Read the model definition and answer for the solid it produces. Units are mm, in the model's axes. Face numbers are marked on the shaded views. A direction names the side the tool comes from. Round coordinates to 2 decimals unless told otherwise and drop trailing zeros. Write each loop counter-clockwise with the first axis right and the second up, starting at its lowest first coordinate (ties: lowest second). Pieces come first, ordered by that corner, then holes. Notation, with made-up numbers: (62.5, -8.5) - (89.5, -8.5) arc R14 cw to (89.5, 0.5) - close; hole circle Ø1 at (17, -12). An arc over 180 degrees is marked (long way). Answer as CSV lines item,"result". Start each with the question number.
1) Find section A-A on x = -2. Determine the outline of the cut face in (y, z), then the cut area to 3 significant figures.
2) Which of the six approach directions +Z, -Z, +X, -X, +Y, -Y give full straight-line access (tool end or side, diameter ignored) to the marked faces 1 and 2?
3) Each of these flat-tipped pins is pushed along its axis until it touches: pin 1 (5.5 mm diameter, centred on x = 21.04, z = 663.49, fed in from -Y); pin 2 (2.5 mm diameter, centred on y = 33.5, z = 640, fed in from -X); pin 3 (2 mm diameter, centred on x = -23.5, z = -74.5, fed in from +Y); pin 4 (4.5 mm diameter, centred on x = -21.04, z = 663.49, fed in from +Y). Where does it stop, or does it pass through?
4) Consider line 1 along Y through (x, z) = (14, 189.5); line 2 along Y through (x, z) = (-27, 585); line 3 along Z through (x, y) = (-16.5, 13). Determine where each line is inside the solid, lowest interval first.
5) Find section B-B on z = -339. Determine the outline of the cut face in (x, y), then the cut area to 3 significant figures.
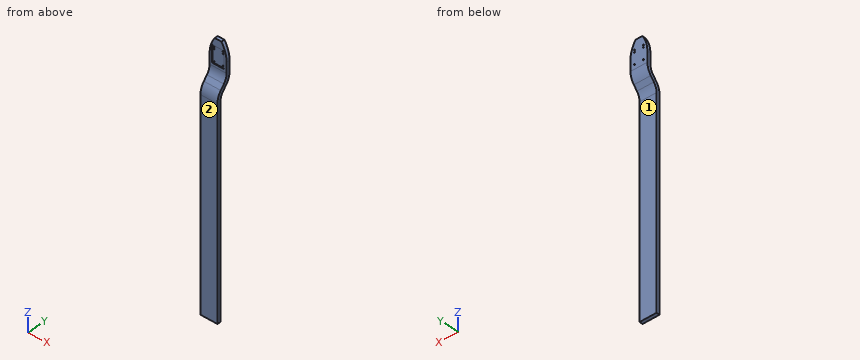
Autodesk Inventor part; units mm, degrees
ref_plane "YZ Plane" through (0, 0, 0) normal (1, 0, 0) x (0, 1, 0)
ref_plane "XZ Plane" through (0, 0, 0) normal (0, 1, 0) x (-1, 0, 0)
ref_plane "XY Plane" through (0, 0, 0) normal (0, 0, 1) x (1, 0, 0)
sketch "Sketch1" plane through (0, 0, 0) normal (0, 1, 0) x (-1, 0, 0)
  line L0 (-40, 482.6) -> (-40, -482.6)
  line L1 (-40, -482.6) -> (40, -482.6)
  line L2 (40, -482.6) -> (40, 482.6)
  line L3 (40, 482.6) -> (-40, 482.6)
  line L4 (-40, 482.6) -> (40, -482.6) construction
  line L5 (-40, -482.6) -> (40, 482.6) construction
  point P0 (0, 0)
  dimension "d0" = 965.2
  dimension "d1" = 80
extrude "Extrusion1" add sketch "Sketch1" against normal blind 15.5448
ref_plane "Work Plane1" through (0, 0, 482.6) normal (1, 0, 0) x (0, 1, 0)
sketch "Sketch2" plane through (0, 0, 482.6) normal (1, 0, 0) x (0, 1, 0)
  line L0 (0, -965.2) -> (0, 0)
  line L1 (0, -965.2) -> (-15.5448, -965.2)
  line L2 (-15.5448, 0) -> (-15.5448, -965.2)
  line L3 (0, 0) -> (-15.5448, 0)
  line L4 (41.9902, -1050.1493) -> (41.9902, -1135.1493)
  line L5 (57.0671, -1050.1493) -> (57.0671, -1135.1493)
  line L6 (57.0671, -1135.1493) -> (41.9902, -1135.1493)
  line L7 (41.9902, -1092.6493) -> (57.0671, -1092.6493) construction
  line L8 (-15.5448, 0) -> (-15.5448, -965.2) construction
  line L9 (-15.5448, -965.2) -> (-15.5448, -1004.6981) construction
  line L10 (-15.5448, -1004.6981) -> (41.9902, -1021.6042) construction
  line L11 (41.9902, -1021.6042) -> (41.9902, -1050.1493) construction
  spline S0 degree 3 poles (-15.5448, -965.2) (-15.5448, -1004.6981) (41.9902, -1021.6042) (41.9902, -1050.1493) knots 1 1 1 1 2 2 2 2
  line L12 (57.0671, -1050.1493) -> (57.0671, -1021.6042) construction
  line L13 (57.0671, -1021.6042) -> (0, -1003.1803) construction
  line L14 (0, -965.2) -> (0, 0) construction
  line L15 (0, -1003.1803) -> (0, -965.2) construction
  spline S1 degree 3 poles (57.0671, -1050.1493) (57.0671, -1021.6042) (0, -1003.1803) (0, -965.2) knots 1 1 1 1 2 2 2 2
  point P0 (0, -482.6)
  dimension "d4" = 85
  dimension "d5" = 15.0769
sketch "Sketch3" plane through (0, 0, 482.6) normal (1, 0, 0) x (0, 1, 0)
  line L0 (0, 0) -> (0, -965.2)
  line L1 (0, 0) -> (-15.5448, 0)
  line L2 (-15.5448, -965.2) -> (-15.5448, 0)
  line L3 (0, -965.2) -> (-15.5448, -965.2)
  arc A0 (2.1293, 48.5593) -> (-15.5448, 0) centre (60, 0) ccw
  arc A1 (14.0373, 38.5673) -> (0, 0) centre (60, 0) ccw
  line L4 (2.1293, 48.5593) -> (18.199, 67.7104)
  line L5 (0, 0) -> (-15.5448, 0) construction
  line L6 (2.1293, 48.5593) -> (14.0373, 38.5673) construction
  line L7 (14.0373, 38.5673) -> (30.107, 57.7184)
  arc A2 (18.199, 67.7104) -> (32.2363, 106.2776) centre (-27.7637, 106.2776) ccw
  arc A3 (30.107, 57.7184) -> (47.7811, 106.2776) centre (-27.7637, 106.2776) ccw
  line L8 (32.2363, 106.2776) -> (32.2363, 233.2776)
  line L9 (32.2363, 233.2776) -> (47.7811, 233.2776)
  line L10 (47.7811, 233.2776) -> (47.7811, 106.2776)
  line L11 (30.107, 57.7184) -> (18.199, 67.7104) construction
  line L12 (32.2363, 106.2776) -> (47.7811, 106.2776) construction
  point P0 (0, -482.6)
  dimension "d17" = 127
  dimension "d18" = 140
  dimension "d19" = 60
  dimension "d21" = 140
  dimension "d22" = 25
extrude "Extrusion2" add sketch "Sketch3" along normal up to surface (80 mm away) from surface at -40 contours L1 A0 L4 A2 L8 L9 L10 A3 L7 A1
sketch "Sketch9" plane through (-40, 47.7811, 588.8776) normal (0, 1, 0) x (1, 0, 0)
  line L0 (0, -127) -> (0, 0) construction
  line L1 (0, 0) -> (0, -127) construction
  line L2 (80, -127) -> (80, 0) construction
  line L3 (0, -127) -> (0, -49.1262)
  line L4 (80, 0) -> (80, -127)
  line L5 (80, -49.1262) -> (80, -127)
  arc A0 (0, -49.1262) -> (24.125, -127) centre (137.7482, -49.1262) ccw
  arc A1 (55.875, -127) -> (80, -49.1262) centre (-57.7482, -49.1262) ccw
  line L6 (24.125, -127) -> (55.875, -127)
  line L7 (0, -127) -> (80, -127)
  line L8 (55.875, -127) -> (80, -127)
  line L9 (80, -127) -> (80, -49.1262)
  line L10 (0, -127) -> (24.125, -127)
  line L11 (55.875, -127) -> (80, -127)
  line L12 (24.125, -127) -> (0, -127)
  point P0 (40, 588.8776)
  dimension "d41" = 31.75
sketch "Sketch10" plane through (-40, 47.7811, 588.8776) normal (0, 1, 0) x (1, 0, 0)
  line L0 (11.425, -92.075) -> (68.575, -92.075) construction
  line L1 (68.575, -92.075) -> (68.575, -12.7) construction
  line L2 (68.575, -12.7) -> (11.425, -12.7) construction
  line L3 (11.425, -12.7) -> (11.425, -92.075) construction
  line L4 (11.425, -92.075) -> (68.575, -12.7) construction
  line L5 (68.575, -92.075) -> (11.425, -12.7) construction
  line L6 (12.6315, -90.043) -> (67.3685, -90.043)
  line L7 (67.3685, -90.043) -> (67.3685, -14.732)
  line L8 (67.3685, -14.732) -> (12.6315, -14.732)
  line L9 (12.6315, -14.732) -> (12.6315, -90.043)
  line L10 (12.6315, -90.043) -> (67.3685, -14.732) construction
  line L11 (67.3685, -90.043) -> (12.6315, -14.732) construction
  line L12 (18.965, -84.1375) -> (61.035, -84.1375) construction
  line L13 (61.035, -84.1375) -> (61.035, -20.6375) construction
  line L14 (61.035, -20.6375) -> (18.965, -20.6375) construction
  line L15 (18.965, -20.6375) -> (18.965, -84.1375) construction
  line L16 (18.965, -84.1375) -> (61.035, -20.6375) construction
  line L17 (61.035, -84.1375) -> (18.965, -20.6375) construction
  line L18 (18.965, -84.1375) -> (61.035, -84.1375) construction
  line L19 (61.035, -84.1375) -> (61.035, -74.6125) construction
  line L20 (61.035, -74.6125) -> (18.965, -74.6125) construction
  line L21 (18.965, -74.6125) -> (18.965, -84.1375) construction
  line L22 (68.575, -12.7) -> (80, -12.7) construction
  line L23 (11.425, -12.7) -> (0, -12.7) construction
  line L24 (0, -127) -> (0, 0) construction
  line L25 (80, -127) -> (80, 0)
  line L26 (0, 0) -> (80, 0)
  point P0 (40, 588.8776)
  point P1 (40, -52.3875)
  dimension "d33" = 57.15
  dimension "d34" = 79.375
  dimension "d35" = 54.737
  dimension "d36" = 75.311
  dimension "d37" = 42.07
  dimension "d38" = 63.5
  dimension "d39" = 9.525
  dimension "d40" = 12.7
extrude "Extrusion7" cut sketch "Sketch9" against normal through all
hole "Hole1" at (-21.035, 47.7811, 673.0151) at (-21.035, 47.7811, 663.4901) at (21.035, 47.7811, 673.0151) at (21.035, 47.7811, 663.4901) at (21.035, 47.7811, 609.5151) at (-21.035, 47.7811, 609.5151) direction (0, -1, 0) diameter 4.7625 end through all
sketch "Sketch11" plane through (-40, 32.2363, 588.8776) normal (0, -1, 0) x (1, 0, 0)
  line L0 (11.425, 92.075) -> (68.575, 92.075) construction
  line L1 (11.425, 12.7) -> (11.425, 92.075) construction
  line L2 (68.575, 92.075) -> (68.575, 12.7) construction
  line L3 (11.425, 12.7) -> (68.575, 12.7)
  line L4 (68.575, 12.7) -> (68.575, 92.075)
  line L5 (68.575, 92.075) -> (11.425, 92.075)
  line L6 (11.425, 92.075) -> (11.425, 12.7)
  line L7 (11.425, 12.7) -> (68.575, 92.075) construction
  line L8 (68.575, 12.7) -> (11.425, 92.075) construction
  point P0 (40, -588.8776)
  point P1 (40, 52.3875)
extrude "Extrusion8" cut sketch "Sketch11" against normal blind 3
properties part number "Metal Middle" material "Aluminum 6061"
Check values:
1,outline,"(-15.54, -482.6) - (0, -482.6) - (0, 482.6) arc R60 cw to (14.04, 521.17) - (30.11, 540.32) arc R75.54 ccw to (47.78, 588.88) - (47.78, 715.88) - (32.24, 715.88) - (32.24, 680.95) - (35.24, 680.95) - (35.24, 601.58) - (32.24, 601.58) - (32.24, 588.88) arc R60 cw to (18.2, 550.31) - (2.13, 531.16) arc R75.54 ccw to (-15.54, 482.6) - close"
1,area,"18,600 mm^2"
2,face 1,"-Z, +X, -X, +Y"
2,face 2,"+Z, -Z, +X, -X, -Y"
3,pin 1,"stops at y = 35.24"
3,pin 2,"stops at x = -40"
3,pin 3,"stops at y = 0"
3,pin 4,"passes through"
4,line 1,"y = -15.54 to 0"
4,line 2,"y = 32.11 to 47.68"
4,line 3,"z = 519.9 to 544.11"
5,outline,"(-40, -15.54) - (40, -15.54) - (40, 0) - (-40, 0) - close"
5,area,"1,240 mm^2"
